Here's the drawing with two shaded views (mm, measured from the low corner). I have some questions. Round coordinates to 2 decimals unless told otherwise and drop trailing zeros. Loops run counter-clockwise (first coordinate to the right, second up) from the corner with the lowest first, then second, coordinate; pieces in that order, holes last.
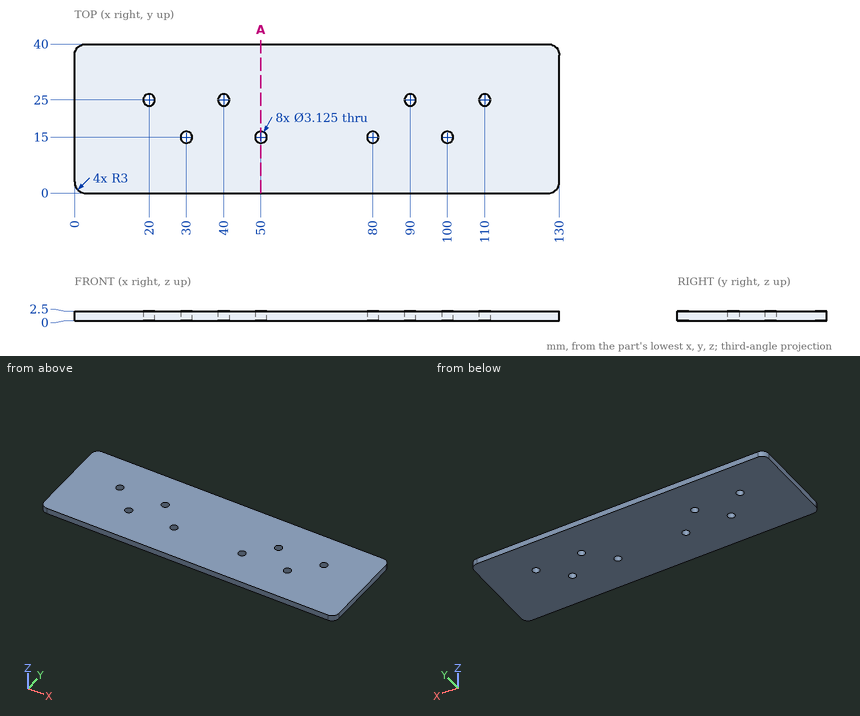
Item 1: If we section it at A-A, the plane x = 50: Please give me the cut outline in (y, z), then the cut area to 3 significant figures.
Results list:
outline: (0, 0) - (13.44, 0) - (13.44, 2.5) - (0, 2.5) - close; (16.56, 0) - (40, 0) - (40, 2.5) - (16.56, 2.5) - close
area: 92.2 mm2
Item 2: Will this pin go through, and if not, where does the flat tip stop? pin 1 (2.5 mm diameter, centred on x = 90, y = 25, fed in from -Z).
Results list:
pin 1: passes through
Item 3: If I drill on line 1 along Y through (x, z) = (80, 1.1); line 2 along Y through (x, z) = (20, 0.9), over which ranges is the centre line in solid material (lowest first)?
Results list:
line 1: y = 0 to 13.44, 16.56 to 40
line 2: y = 0 to 23.44, 26.56 to 40
